Design review of the part built by this model. Coordinates are the model's own, in mm. A direction names the side the tool comes from. Round coordinates to 2 decimals unless told otherwise and drop trailing zeros. Order: outer loops, then holes, each group sorted by start corner. A loop starts at its lowest first (then second) coordinate and runs counter-clockwise, first axis right, second up. Notation, with made-up numbers: (78, 70.25) - (93, 70.25) arc R18 cw to (93, 89.25) - close; hole circle Ø6 at (57, 53.5). An arc over 180 degrees is marked (long way). Use CSV: the item, a comma, the result in double quotes.
from build123d import *

# Parameters (mm, degrees)
F0_W     = 1.5
F0_H     = 1.5
F1_DEPTH = 0.75


with BuildPart() as f1:
    # F0 (on Front) → F1 (new body, symmetric)
    with BuildSketch(Plane.XZ):
        Polygon((-54.428298, -57.24404), (-53.57977, -58.092568), (-50.37977, -54.892568), (-50.37977, -48.592568), (-49.77977, -47.992568), (-49.77977, -43.974031), (-49.77977, -42.474031), (-49.77977, -18.689784), (-49.77977, -17.189784), (-49.77977, -13.796059), (-49.77977, -12.296059), (-49.77977, 6.816904), (-49.77977, 8.316904), (-49.77977, 29.209403), (-49.77977, 30.709403), (-49.77977, 35.607432), (-51.27977, 35.607432), (-51.27977, -47.992568), (-51.87977, -48.592568), (-51.87977, -54.695512), align=None)
        with Locations((-49.02977, -43.224031)):
            Rectangle(F0_W, F0_H)
        with Locations((-49.02977, -17.939784)):
            Rectangle(F0_W, F0_H)
        with Locations((-49.02977, 29.959403)):
            Rectangle(F0_W, F0_H)
        with Locations((-49.02977, 7.566904)):
            Rectangle(F0_W, F0_H)
    extrude(amount=F1_DEPTH, both=True)


solid = f1.part
1) We need section A-A (y = 0.05). Give the boundary of the cut face in (x, z), then the cut area to 3 significant figures.
Data:
outline,"(-54.43, -57.24) - (-53.58, -58.09) - (-50.38, -54.89) - (-50.38, -48.59) - (-49.78, -47.99) - (-49.78, -43.97) - (-48.28, -43.97) - (-48.28, -42.47) - (-49.78, -42.47) - (-49.78, -18.69) - (-48.28, -18.69) - (-48.28, -17.19) - (-49.78, -17.19) - (-49.78, 6.82) - (-48.28, 6.82) - (-48.28, 8.32) - (-49.78, 8.32) - (-49.78, 29.21) - (-48.28, 29.21) - (-48.28, 30.71) - (-49.78, 30.71) - (-49.78, 35.61) - (-51.28, 35.61) - (-51.28, -47.99) - (-51.88, -48.59) - (-51.88, -54.7) - close"
area,"149 mm2"
2) We need section B-B (z = 16.5). Give the boundary of the cut face in (x, y).
Data:
outline,"(-51.28, -0.75) - (-49.78, -0.75) - (-49.78, 0.75) - (-51.28, 0.75) - close"
3) To check wall thickness, follow L1, parallel to Z at x = -49, y = -0.3; L2, parallel to X at y = 0.65, z = 14; L3, parallel to Z at x = -52.25, y = -0.1. State the ranges of each line that lie inside material, in increasing order. Write a range as from..to.
Data:
L1,"z = -43.97..-42.47, -18.69..-17.19, 6.82..8.32, 29.21..30.71"
L2,"x = -51.28..-49.78"
L3,"z = -56.76..-55.07"
4) For faces 1 (the face through (-49, 0, 6.817)), 2 (the face through (-48.28, 0, 30)), 3 (the face through (-51.88, 0, -52)), 4 (the face through (-49, 0, -43.974)), 5 (the face through (-49, 0, 30.709)), list the 3-axis set-ups (+Z, -Z, +X, -X, +Y, -Y) from which the entire face can be reached by the end or side of a thin tool; tool diameter is ignored.
Data:
face 1,"+X, +Y, -Y"
face 2,"+Z, -Z, +X, +Y, -Y"
face 3,"+Z, -X, +Y, -Y"
face 4,"-Z, +X, +Y, -Y"
face 5,"+Z, +X, +Y, -Y"
5) Insertion check: pin 1 Ø0.8 at (y, z) = (0, -51) entering from +X; pin 2 Ø0.8 at (x, y) = (-49, 0) entering from +Z; pin 3 Ø0.8 at (x, y) = (-49.5, 0) entering from -Z. Each pin has a flat end and moves straight along its axis. Give the tip position at first contact, or say it passes through.
Data:
pin 1,"stops at x = -50.38"
pin 2,"stops at z = 30.71"
pin 3,"stops at z = -48.11"
